Geometry check sheet. Reference: the model listing, model coordinates, mm. A direction names the side the tool comes from. Round coordinates to 2 decimals unless told otherwise and drop trailing zeros. Write each loop counter-clockwise with the first axis right and the second up, starting at its lowest first coordinate (ties: lowest second). Pieces come first, ordered by that corner, then holes. Notation, with made-up numbers: (59.25, 31.5) -> (101.25, 31.5) arc R13 cw to (101.25, 36.5) -> close; hole circle Ø4 at (14, -36). An arc over 180 degrees is marked (long way). One line per question, with ' | ' between items.
```python
from build123d import *

# Parameters (mm, degrees)
SKETCH_1_W          = 15
SKETCH_1_H          = 15
EXTRUDE_1_DEPTH     = 5
SKETCH_2_R          = 1.5
SKETCH_2_R_2        = 1.25
SKETCH_2_R_3        = 2.8
SKETCH_2_R_4        = 1
CUT_EXTRUDE_1_DEPTH = 5
FILLET_1_R          = 1.5
SKETCH_4_R          = 1.5
EXTRUDE_2_DEPTH     = 2
SKETCH_5_R          = 2
CUT_EXTRUDE_2_DEPTH = 5


with BuildPart() as part:
    # 草图1 → 凸台-拉伸1 (new body)
    with BuildSketch(Plane(origin=(0, 0, 0), x_dir=(1, 0, 0), z_dir=(0, 1, 0))):
        Polygon((30, 10), (-30, 10), (-30, 5), (-30, -10), (30, -10), align=None)
        with Locations((-37.5, -2.5)):
            Rectangle(SKETCH_1_W, SKETCH_1_H)
    extrude(amount=EXTRUDE_1_DEPTH)

    # 草图2 → 切除-拉伸1 (cut)
    with BuildSketch(Plane(origin=(0, 5, 0), x_dir=(1, 0, 0), z_dir=(0, 1, 0))):
        with Locations(Location((8.5, 0, 0), (0, 0, 270))):
            Circle(SKETCH_2_R)
        with Locations(Location((-8.5, 0, 0), (0, 0, 90))):
            Circle(SKETCH_2_R)
        with Locations(Location((0, 0, 0), (0, 0, 270))):
            Circle(SKETCH_2_R_2)
        with Locations(Location((20, 0, 0), (0, 0, 270))):
            Circle(SKETCH_2_R_3)
        with Locations(Location((-20, 0, 0), (0, 0, 90))):
            Circle(SKETCH_2_R_3)
        with Locations(Location((20, 8, 0), (0, 0, 270))):
            Circle(SKETCH_2_R_2)
        with Locations(Location((28, 0, 0), (0, 0, 270))):
            Circle(SKETCH_2_R_2)
        with Locations(Location((-28, 0, 0), (0, 0, 90))):
            Circle(SKETCH_2_R_2)
        with Locations(Location((-20, 8, 0), (0, 0, 90))):
            Circle(SKETCH_2_R_2)
        with Locations(Location((-37.5, -2.5, 0), (0, 0, 270))):
            Circle(SKETCH_2_R)
        with Locations(Location((-32, -2.5, 0), (0, 0, 270))):
            Circle(SKETCH_2_R_4)
        with Locations(Location((-37.5, -8, 0), (0, 0, 270))):
            Circle(SKETCH_2_R_4)
        with Locations(Location((-43, -2.5, 0), (0, 0, 270))):
            Circle(SKETCH_2_R_4)
        with Locations(Location((-37.5, 3, 0), (0, 0, 270))):
            Circle(SKETCH_2_R_4)
    extrude(amount=-CUT_EXTRUDE_1_DEPTH, mode=Mode.SUBTRACT)

    # 圆角1
    fillet_1_edges = [part.edges().sort_by_distance(p)[0] for p in [
        (-30, 2.5, -5),
        (-45, 2.5, -5),
        (-30, 2.5, -10),
        (30, 2.5, -10),
    ]]
    fillet(fillet_1_edges, radius=FILLET_1_R)

    # 草图4 → 凸台-拉伸2 (add)
    with BuildSketch(Plane.XY.offset(10)):
        with Locations(Location((20, 2.5, 0), (0, 0, 180))):
            Circle(SKETCH_4_R)
        with Locations(Location((-20, 2.5, 0), (0, 0, 180))):
            Circle(SKETCH_4_R)
    extrude(amount=EXTRUDE_2_DEPTH)

    # 草图5 → 切除-拉伸2 (cut)
    with BuildSketch(Plane(origin=(0, 0, -10), x_dir=(-1, 0, 0), z_dir=(0, 0, -1))):
        with Locations((-20, 2.5)):
            Circle(SKETCH_5_R)
        with Locations(Location((20, 2.5, 0), (0, 0, 180))):
            Circle(SKETCH_5_R)
    extrude(amount=-CUT_EXTRUDE_2_DEPTH, mode=Mode.SUBTRACT)


solid = part.part
```
(1) Draft check along Z on faces 4 (the cylindrical face through (-18.5, 2.43, 10.99)), 5 (the flat face through (-8, 2, 10)), 6 (the cylindrical face through (-36.51, 2.54, -3.13)). Enter one of: +Z half, -Z half, draft (parallel to the pull), parting line (faces both ways), or undercut.
Resolved:
face 4: draft | face 5: +Z half | face 6: undercut
(2) Sectioned sample at A-A on x = 0. Record the cut outline in (y, z).
Resolved:
outline: (0, -10) -> (5, -10) -> (5, -1.25) -> (0, -1.25) -> close; (0, 1.25) -> (5, 1.25) -> (5, 10) -> (0, 10) -> close
(3) Access from +Z, -Z, +X, -X, +Y, -Y to the whole of each face (thin tool, end or side, straight path). Record for faces 1 (the flat face through (-20, 2, -5)), 2 (the flat face through (-30, 2, -8)), 3 (the cylindrical face through (21.5, 2.43, 10.99)).
Resolved:
face 1: -Z | face 2: -Z, -X, +Y, -Y | face 3: +Z
(4) Sectioned sample at B-B on x = -37.5. Record the cut outline in (y, z).
Resolved:
outline: (0, -5) -> (5, -5) -> (5, -4) -> (0, -4) -> close; (0, -2) -> (5, -2) -> (5, 1) -> (0, 1) -> close; (0, 4) -> (5, 4) -> (5, 7) -> (0, 7) -> close; (0, 9) -> (5, 9) -> (5, 10) -> (0, 10) -> close
(5) Sectioned sample at D-D on z = 7.75. Record the cut outline in (x, y), then the cut area to 3 significant figures.
Resolved:
outline: (-45, 0) -> (-38.47, 0) -> (-38.47, 5) -> (-45, 5) -> close; (-36.53, 0) -> (30, 0) -> (30, 5) -> (-36.53, 5) -> close | area: 365 mm2
(6) Material ranges on line 1 (X direction, y = 0.65, z = -8); line 2 (X direction, y = 1.8, z = 2.5); line 3 (X direction, y = 3.05, z = -7.5), recorded low to high.
Resolved:
line 1: x = -30 to -21.25, -18.75 to 18.75, 21.25 to 30 | line 2: x = -45 to -44, -42 to -39, -36 to -33, -31 to -21.26, -18.74 to 18.74, 21.26 to 30 | line 3: x = -30 to -21.92, -18.08 to 18.08, 21.92 to 30
(7) Go/stop test with flat-tipped pins: pin 1 (3 mm diameter, centred on x = 20, y = 2.5, fed in from -Z); pin 2 (1 mm diameter, centred on y = 3, z = -7, fed in from -X). Record where each tip stops, or that it passes through.
Resolved:
pin 1: stops at z = -5 | pin 2: stops at x = -30
(8) Sectioned sample at C-C on z = 0.25. Count the separate pieces of the cut face and the enclosed holes in it, then the cut area to 3 significant figures.
Resolved:
separate pieces: 8 | enclosed holes: 0 | area: 253 mm2
